```python
from build123d import *

# Parameters (mm, degrees)
SKETCH_1_W          = 20
SKETCH_1_H          = 105
SKETCH_1_W_2        = 65
SKETCH_1_H_2        = 45
SKETCH_1_W_3        = 7
SKETCH_1_H_3        = 59
EXTRUDE_2_DEPTH     = 3
SKETCH_1_5_W        = 97
SKETCH_1_5_H        = 37
CUT_EXTRUDE_1_DEPTH = 126.584632818
SKETCH_1_6_R        = 1.25
SKETCH_1_6_R_2      = 1.6
CUT_EXTRUDE_3_DEPTH = 126.584632818
SKETCH_1_7_R        = 2
CUT_EXTRUDE_4_DEPTH = 1.5


with BuildPart() as part:
    # Sketch 1 → Extrude 2 (new body)
    with BuildSketch(Plane(origin=(0, 0, 0), x_dir=(1, 0, 0), z_dir=(0, 1, 0))):
        with Locations((7.5, -20)):
            Rectangle(SKETCH_1_W, SKETCH_1_H)
        with Locations((92.5, -20)):
            Rectangle(SKETCH_1_W, SKETCH_1_H)
        with Locations((50, -20)):
            Rectangle(SKETCH_1_W_2, SKETCH_1_H_2)
        with Locations((21, -20)):
            Rectangle(SKETCH_1_W_3, SKETCH_1_H_3)
        with Locations((79, -20)):
            Rectangle(SKETCH_1_W_3, SKETCH_1_H_3)
    extrude(amount=EXTRUDE_2_DEPTH)

    # Sketch 1_5 → Cut-Extrude 1 (cut, through all)
    with BuildSketch(Plane(origin=(0, 0, 0), x_dir=(1, 0, 0), z_dir=(0, 1, 0))):
        with Locations((50, -20)):
            Rectangle(SKETCH_1_5_W, SKETCH_1_5_H)
    extrude(amount=CUT_EXTRUDE_1_DEPTH, mode=Mode.SUBTRACT)

    # Sketch 1_6 → Cut-Extrude 3 (cut, through all)
    with BuildSketch(Plane(origin=(0, 0, 0), x_dir=(1, 0, 0), z_dir=(0, 1, 0))):
        with Locations(Location((21, 6, 0), (0, 0, 270))):
            Circle(SKETCH_1_6_R)
        with Locations(Location((79, 6, 0), (0, 0, 270))):
            Circle(SKETCH_1_6_R)
        with Locations(Location((79, -46, 0), (0, 0, 270))):
            Circle(SKETCH_1_6_R)
        with Locations(Location((21, -46, 0), (0, 0, 270))):
            Circle(SKETCH_1_6_R)
        with Locations(Location((7.5, 21.35, 0), (0, 0, 270))):
            Circle(SKETCH_1_6_R_2)
        with Locations(Location((92.5, 21.35, 0), (0, 0, 270))):
            Circle(SKETCH_1_6_R_2)
        with Locations(Location((92.5, -61.35, 0), (0, 0, 270))):
            Circle(SKETCH_1_6_R_2)
        with Locations(Location((7.5, -61.35, 0), (0, 0, 270))):
            Circle(SKETCH_1_6_R_2)
    extrude(amount=CUT_EXTRUDE_3_DEPTH, mode=Mode.SUBTRACT)

    # Sketch 1_7 → Cut-Extrude 4 (cut)
    with BuildSketch(Plane(origin=(0, 0, 0), x_dir=(1, 0, 0), z_dir=(0, 1, 0))):
        with Locations(Location((21, 6, 0), (0, 0, 270))):
            Circle(SKETCH_1_7_R)
        with Locations(Location((79, 6, 0), (0, 0, 270))):
            Circle(SKETCH_1_7_R)
        with Locations(Location((79, -46, 0), (0, 0, 270))):
            Circle(SKETCH_1_7_R)
        with Locations(Location((21, -46, 0), (0, 0, 270))):
            Circle(SKETCH_1_7_R)
    extrude(amount=CUT_EXTRUDE_4_DEPTH, mode=Mode.SUBTRACT)


solid = part.part
```
Work out the finished part from the listing and answer in its coordinate system (mm). A direction names the side the tool comes from. Round coordinates to 2 decimals unless told otherwise and drop trailing zeros. Write each loop counter-clockwise with the first axis right and the second up, starting at its lowest first coordinate (ties: lowest second). Pieces come first, ordered by that corner, then holes. Notation, with made-up numbers: (5.5, 39.25) -> (11.5, 39.25) arc R29 ccw to (11.5, 70.25) -> close; hole circle Ø9 at (67, 32.25). An arc over 180 degrees is marked (long way). Write each question's results on one line, items separated by ' | '.
Q1. Which of the six approach directions +Z, -Z, +X, -X, +Y, -Y give full straight-line access (tool end or side, diameter ignored) to faces 4 (the cylindrical face through (81, 1, -6)), 5 (the flat face through (7, 1, -32.5)), 6 (the flat face through (75.5, 1, -6)), 7 (the flat face through (82.5, 1, 61)), 8 (the flat face through (98.5, 1, 20))?
Data:
face 4: -Y | face 5: -Z, +X, -X, +Y, -Y | face 6: -Z, +Y, -Y | face 7: +Z, +Y, -Y | face 8: +Y, -Y
Q2. Straight lines are drawn through the part: line 1 along Z through (x, y) = (92.5, 1.75); line 2 along X through (y, z) = (0.95, 46); line 3 along Z through (x, y) = (67, 1.15). For each, find the intervals that lie inside material, in ascending order. Write a range as [from, to].
Data:
line 1: [-32.5, -22.95], [-19.75, 1.5], [38.5, 59.75], [62.95, 72.5] | line 2: [-2.5, 19], [23, 24.5], [75.5, 77], [81, 102.5] | line 3: [-2.5, 1.5], [38.5, 42.5]
Q3. Section B-B, the plane x = 92.5 is taken. Write down the section's boundary in (y, z), then the cut area to 3 significant figures.
Data:
outline: (0, -32.5) -> (3, -32.5) -> (3, -22.95) -> (0, -22.95) -> close; (0, -19.75) -> (3, -19.75) -> (3, 1.5) -> (0, 1.5) -> close; (0, 38.5) -> (3, 38.5) -> (3, 59.75) -> (0, 59.75) -> close; (0, 62.95) -> (3, 62.95) -> (3, 72.5) -> (0, 72.5) -> close | area: 185 mm^2
Q4. Section D-D, the plane z = 13.5 is taken. Write down the section's boundary in (x, y), then the cut area to 3 significant figures.
Data:
outline: (-2.5, 0) -> (1.5, 0) -> (1.5, 3) -> (-2.5, 3) -> close; (98.5, 0) -> (102.5, 0) -> (102.5, 3) -> (98.5, 3) -> close | area: 24.0 mm^2
Q5. Flat-ended cylindrical pins translate along their axes: P1, Ø0.9, axis at x = 79.5, y = 1.5, coming from the +Z side; P2, Ø1, axis at x = 43, y = 1, coming from the +Z side. Find the tip coordinate at first contact, or state that the pin passes through.
Data:
P1: z = 49.5 | P2: z = 42.5
Q6. Section C-C, the plane x = 32.5 is taken. Write down the section's boundary in (y, z).
Data:
outline: (0, -2.5) -> (3, -2.5) -> (3, 1.5) -> (0, 1.5) -> close; (0, 38.5) -> (3, 38.5) -> (3, 42.5) -> (0, 42.5) -> close
Q7. Determine the mould class of faces 1 (the flat face through (92, 1, -32.5)), 2 (the flat face through (102.5, 1, 21)), 3 (the flat face through (1.5, 1, 20)) for opening direction X: released by +X, released by -X, zero draft, split by the parting line, or undercut.
Data:
face 1: zero draft | face 2: released by +X | face 3: undercut
Q8. Section A-A, the plane z = 61.35 is taken. Write down the section's boundary in (x, y), then the cut area to 3 significant figures.
Data:
outline: (-2.5, 0) -> (5.9, 0) -> (5.9, 3) -> (-2.5, 3) -> close; (9.1, 0) -> (17.5, 0) -> (17.5, 3) -> (9.1, 3) -> close; (82.5, 0) -> (90.9, 0) -> (90.9, 3) -> (82.5, 3) -> close; (94.1, 0) -> (102.5, 0) -> (102.5, 3) -> (94.1, 3) -> close | area: 101 mm^2
